Autodesk Inventor part; units mm, degrees
ref_plane "Work Plane1" through (24.6957, 5, 24.6957) normal (0.7071068, 0, 0.7071068) x (0.7071068, 0, -0.7071068)
ref_plane "YZ Plane" through (0, 0, 0) normal (1, 0, 0) x (0, 1, 0)
ref_plane "XZ Plane" through (0, 0, 0) normal (0, 1, 0) x (-1, 0, 0)
sketch "Sketch1" plane through (0, 0, 0) normal (0, 1, 0) x (-1, 0, 0)
  line L0 (101.6, -101.6) -> (-101.6, -101.6)
  line L1 (-101.6, -101.6) -> (-101.6, 101.6)
  line L2 (-101.6, 101.6) -> (101.6, 101.6)
  line L3 (101.6, 101.6) -> (101.6, -101.6)
  line L4 (96.6, -96.6) -> (-96.6, -96.6)
  line L5 (-96.6, -96.6) -> (-96.6, 96.6)
  line L6 (-96.6, 96.6) -> (96.6, 96.6)
  line L7 (96.6, 96.6) -> (96.6, -96.6)
  line L8 (101.6, 101.6) -> (-40.4, 101.6)
  circle A0 centre (0, 0) radius 88.9
  circle A1 centre (0, 0) radius 109.3376
  line L9 (-40.4, 101.6) -> (-101.6, 40.4)
  line L10 (-45.4, 101.6) -> (-101.6, 45.4)
  line L11 (96.6, 96.6) -> (96.6, 101.6)
  line L12 (-45.4, 101.6) -> (-35.4, 101.6)
  line L13 (-35.4, 101.6) -> (-35.4, 96.6)
  line L14 (-35.4, 96.6) -> (-45.4, 96.6)
  line L15 (-45.4, 96.6) -> (-45.4, 101.6)
  line L16 (-45.4, 101.6) -> (-43.114, 101.6)
  line L17 (-43.114, 101.6) -> (-43.114, 96.6)
  line L18 (-43.114, 96.6) -> (-45.4, 96.6)
  line L19 (-45.4, 96.6) -> (-45.4, 101.6)
  line L20 (-96.6, 45.4) -> (-101.6, 45.4)
  line L21 (-101.6, 45.4) -> (-101.6, 43.114)
  line L22 (-101.6, 43.114) -> (-96.6, 43.114)
  line L23 (-96.6, 43.114) -> (-96.6, 45.4)
  point P0 (96.6, 51.2168)
  point P1 (101.6, 40.4)
  point P2 (101.6, -40.4)
  point P3 (96.6, -51.2168)
  point P4 (-96.6, 45.4)
  point P5 (-45.4, 96.6)
  dimension "d0" = 203.2
  dimension "d1" = 203.2
  dimension "d2" = 101.6
  dimension "d3" = 101.6
  dimension "d4" = 5
  dimension "d5" = 5
  dimension "d6" = 5
  dimension "d7" = 5
  dimension "d10" = 142
  dimension "d12" = 61.2
  dimension "d14" = 177.8
  dimension "d15" = 5
  dimension "d16" = 5
  dimension "d17" = 10
  dimension "d86" = 2.286
  dimension "d87" = 2.286
extrude "Extrusion1" add sketch "Sketch1" along normal blind 5 contours L0 A1 L4 L7 L3 | L0 A1 L4 | A1 L7 L3 | L0 L1 A1 L5 L4 | A1 L7 L4 | L4 A1 L5 L9 L6 L7 | A1 L7 L11 L2 L3 | L4 L5 A1 | A1 L6 L7 | L1 L9 L22 L5 A1 | L11 L6 A1 L2 | L6 L13 L2 A1 | L1 L22 A1 | A1 L22 L9 | L22 L9 L5 | L6 L17 L9 L2 L13 | L1 L20 A1 L22 | A1 L20 L9 L22 | L20 A1 L10 L5 | L5 L10 L6 L9 | A1 L17 L2 | L9 L17 A1 | L6 L9 L17 | L1 L2 L10 A1 L6 L5 | L10 A1 L20 | L10 A1 L5 | L5 A1 L6 L10 | L15 A1 L17 L9 | L6 L10 A1 L15 | L17 A1 L15 L2 | L5 L6 A1 | L6 A1 L10 | A1 L10 L15 | A0
sketch "Sketch3" plane through (0, 5, 0) normal (0, 1, 0) x (1, 0, 0)
  circle A0 centre (0, 0) radius 88.9
  line L0 (-101.6, 101.6) -> (-101.6, -101.6)
  line L1 (-101.6, -101.6) -> (101.6, -101.6)
  line L2 (-101.6, 101.6) -> (101.6, 101.6)
  line L3 (101.6, 101.6) -> (101.6, -101.6)
  line L4 (101.6, -101.6) -> (-101.6, -101.6)
  line L5 (-101.6, -101.6) -> (-101.6, 101.6)
  line L6 (-96.6, 96.6) -> (96.6, 96.6)
  line L7 (96.6, 96.6) -> (96.6, -96.6)
  line L8 (96.6, -96.6) -> (-96.6, -96.6)
  line L9 (-96.6, -96.6) -> (-96.6, 96.6)
  line L10 (-101.6, -101.6) -> (40.4, -101.6)
  circle A1 centre (0, 0) radius 109.3376
  line L11 (40.4, -101.6) -> (101.6, -40.4)
  line L12 (101.6, -101.6) -> (101.6, 101.6)
  line L13 (45.4038, -101.6) -> (101.6, -45.4038)
  line L14 (96.6, -45.4) -> (101.6, -45.4038)
  line L15 (45.4, -96.6) -> (45.4038, -101.6)
  line L16 (96.6, -45.4) -> (101.6, -45.4)
  line L17 (101.6, -45.4) -> (101.6, -43.114)
  line L18 (101.6, -43.114) -> (96.6, -43.114)
  line L19 (96.6, -43.114) -> (96.6, -45.4)
  line L20 (45.4038, -101.6) -> (43.1178, -101.6)
  line L21 (43.1178, -101.6) -> (43.1178, -96.6)
  line L22 (43.1178, -96.6) -> (45.4038, -96.6)
  line L23 (45.4038, -96.6) -> (45.4038, -101.6)
  point P0 (45.4038, -101.6)
  point P1 (50.4038, -96.6)
  point P2 (96.6, -50.4038)
  dimension "d28" = 177.8
  dimension "d29" = 5
  dimension "d30" = 5
  dimension "d31" = 5
  dimension "d32" = 5
  dimension "d33" = 142
  dimension "d76" = 5.0038
  dimension "d77" = 5.0038
  dimension "d88" = 2.286
  dimension "d89" = 2.286
extrude "Extrusion3" cut sketch "Sketch3" against normal blind 2 contours L2 A1 L6 L9 L0 | A1 L9 L0 | L2 A1 L6 | A1 L9 L8 L1 L0 | L2 L3 A1 L7 L6 | A1 L8 L21 L11 L1 | L3 L11 L18 L7 A1 | A1 L21 L1 | L11 L21 A1 | L3 L18 A1 | A1 L18 L11
sketch "Sketch4" plane through (0, 5, 0) normal (0, 1, 0) x (1, 0, 0)
  line L0 (101.6, 101.6) -> (-101.6, 101.6)
  line L1 (-101.6, 101.6) -> (-101.6, -101.6)
  line L2 (-101.6, -101.6) -> (101.6, -101.6)
  line L3 (101.6, -101.6) -> (101.6, 101.6)
  circle A0 centre (0, 0) radius 2.5
  line L4 (11.3314, 2.139) -> (-2.139, -11.3314)
  line L5 (0, 0) -> (-5.6569, 5.6569)
  line L6 (-5.6569, -14.8492) -> (-26.163, 5.6569)
  line L7 (-5.6569, 26.163) -> (14.8492, 5.6569)
  circle A1 centre (-5.6569, 5.6569) radius 14
  line L8 (-26.163, 5.6569) -> (-5.6569, 26.163)
  line L9 (14.8492, 5.6569) -> (-5.6569, -14.8492)
  line L10 (-40.3051, 5.6569) -> (-5.6569, 40.3051)
  line L11 (-5.6569, 40.3051) -> (28.9914, 5.6569)
  line L12 (28.9914, 5.6569) -> (-5.6569, -28.9914)
  line L13 (-5.6569, -28.9914) -> (-40.3051, 5.6569)
  line L14 (-22.6451, 9.1747) -> (-9.1747, 22.6451)
  line L15 (-9.1747, 22.6451) -> (-12.7668, 26.2372)
  line L16 (-12.7668, 26.2372) -> (-26.2372, 12.7668)
  line L17 (-26.2372, 12.7668) -> (-22.6451, 9.1747)
  point P0 (9.525, 22.5)
  point P1 (-9.525, -6.5)
  dimension "d37" = 203.2
  dimension "d38" = 203.2
  dimension "d39" = 8
  dimension "d40" = 28
  dimension "d41" = 29
  dimension "d42" = 29
  dimension "d43" = 14.5
  dimension "d44" = 10
  dimension "d45" = 10
  dimension "d46" = 10
  dimension "d47" = 10
  dimension "d48" = 5.08
  dimension "d49" = 9.525
  dimension "d50" = 9.525
  dimension "d55" = 101.6
  dimension "d56" = 101.6
extrude "Extrusion4" cut sketch "Sketch4" against normal blind 1 contours A0 | L4 L9 L6 L8 L7 | L8 L17 L16 L15 | A1 | L10 L11 L12 L13
sketch "Sketch6" plane through (0, 5, 0) normal (0, 1, 0) x (1, 0, 0)
  line L0 (45.4038, -101.6) -> (0, 0)
  line L1 (50.4038, -96.6) -> (45.4038, -101.6)
  line L2 (96.6, -43.114) -> (96.6, 96.6)
  line L3 (101.6, -101.6) -> (101.6, 101.6)
  circle A0 centre (0, 0) radius 34.925
  circle A1 centre (0, 0) radius 33.425
  line L4 (-101.6, 101.6) -> (-101.6, -101.6)
  line L5 (-101.6, -101.6) -> (40.4, -101.6)
  line L6 (-101.6, -101.6) -> (101.6, -101.6)
  line L7 (101.6, 101.6) -> (101.6, -43.114)
  line L8 (101.6, -45.4038) -> (0, 0)
  line L9 (-96.6, -96.6) -> (43.1178, -96.6)
  line L10 (96.6, -43.114) -> (96.6, 96.6)
  line L11 (43.1178, -101.6) -> (-101.6, -101.6)
  line L12 (101.6, -45.4038) -> (96.6, -50.4038)
  line L13 (45.4038, -101.6) -> (101.6, -45.4038)
  line L14 (43.1178, -101.6) -> (101.6, -101.6)
  line L15 (0, 0) -> (101.6, -50.4076)
  line L16 (50.4076, -101.6) -> (0, 0)
  line L17 (43.1694, -96.6) -> (47.9269, -96.6)
  line L18 (96.6, -43.1694) -> (96.6, -47.9269)
  line L19 (40.4, -101.6) -> (101.6, -40.4)
  point P0 (13.6374, -30.5164)
  point P1 (30.5164, -13.6374)
  point P2 (14.2494, -31.8859)
  point P3 (31.2861, -15.5222)
  point P4 (29.9423, -14.8555)
  point P5 (31.8859, -14.2494)
  point P6 (98.2555, -48.7483)
  point P7 (96.6, -47.9269)
  point P8 (47.9269, -96.6)
  point P9 (15.5222, -31.2861)
  point P10 (96.6, -45.4)
  point P11 (45.4, -96.6)
  point P12 (14.8555, -29.9423)
  point P13 (96.6, -45.4)
  point P14 (45.4, -96.6)
  point P15 (45.4, -96.6)
  point P16 (47.089, -94.911)
  point P17 (94.911, -47.089)
  point P18 (96.6, -45.4)
  point P19 (43.8583, -98.1417)
  point P20 (98.1417, -43.8583)
  point P21 (45.4, -96.6)
  point P22 (96.6, -45.4)
  dimension "d71" = 69.85
  dimension "d72" = 66.85
  dimension "d75" = 142
  dimension "d78" = 5.0038
  dimension "d82" = 5.0038
extrude "Extrusion6" add sketch "Sketch6" along normal blind 54.5 contours L0 A0 L16 L19 L17 | L0 A1 L16 A0 | L16 A1 L15 A0 | L15 A0 L8 L18 L19 | A0 L15 A1 L8
fillet "Fillet3" radius 12.7 1 edges at (101.6, 2.5, 101.6)
sketch "Sketch9" plane through (0, 4, 0) normal (0, 1, 0) x (1, 0, 0)
  point P0 (0, 0)
sketch "Sketch10" plane through (0, 5, 0) normal (0, 1, 0) x (1, 0, 0)
  point P0 (0, 0)
ref_plane "Work Plane1" through (24.6957, 5, 24.6957) normal (0.7071068, 0, 0.7071068) x (0.7071068, 0, -0.7071068)
sketch "Sketch15" plane through (0, 5, 0) normal (0, 1, 0) x (1, 0, 0)
  line L0 (13.6374, -30.5164) -> (43.1694, -96.6)
  line L1 (28.4034, -63.5582) -> (-0.6569, -23.9914)
  line L2 (28.9914, 5.6569) -> (-5.6569, -28.9914)
  line L3 (96.6, -43.1694) -> (30.5164, -13.6374)
  line L4 (-5.6569, 40.3051) -> (28.9914, 5.6569)
  line L5 (63.5582, -28.4034) -> (23.9914, 0.6569)
  line L6 (2.3374, -28.0682) -> (28.0682, -2.3374)
  arc A0 (13.6374, -30.5164) -> (30.5164, -13.6374) centre (0, 0) ccw
  line L7 (28.4034, -63.5582) -> (13.6374, -30.5164)
  line L8 (63.5582, -28.4034) -> (30.5164, -13.6374)
  arc A1 (13.6374, -30.5164) -> (30.5164, -13.6374) centre (0, 0) ccw
  dimension "d138" = 5
  dimension "d139" = 5
  dimension "d140" = 5
extrude "Extrusion11" add sketch "Sketch15" along normal up to surface (54.5 mm away) contours L0 L1 L6 L5 L3 A0
sketch "Sketch16" plane through (0, 59.5, 0) normal (0, 1, 0) x (1, 0, 0)
  line L0 (2.3374, -28.0682) -> (28.0682, -2.3374)
  line L1 (9.4085, -20.9971) -> (12.944, -24.5327)
  line L2 (12.944, -24.5327) -> (24.5327, -12.944)
  line L3 (24.5327, -12.944) -> (20.9971, -9.4085)
  line L4 (12.944, -24.5327) -> (24.5327, -12.944)
  line L5 (24.5327, -12.944) -> (28.5592, -16.9706)
  line L6 (28.5592, -16.9706) -> (16.9706, -28.5592)
  line L7 (16.9706, -28.5592) -> (12.944, -24.5327)
  line L8 (12.944, -24.5327) -> (5.3317, -32.145)
  line L9 (28.4034, -63.5582) -> (2.3374, -28.0682)
  line L10 (24.5327, -12.944) -> (32.145, -5.3317)
  line L11 (28.0682, -2.3374) -> (63.5582, -28.4034)
  point P0 (0, 0)
  dimension "d144" = 10
  dimension "d145" = 10
  dimension "d146" = 5
  dimension "d152" = 0
  dimension "d153" = 0
extrude "Extrusion12" cut sketch "Sketch16" against normal up to surface (54.5 mm away)
sketch "Sketch11" plane through (24.6957, 5, 24.6957) normal (0.7071068, 0, 0.7071068) x (0.7071068, 0, -0.7071068)
  line L0 (143.6841, -5) -> (0, -5)
  line L1 (0, -5) -> (0, 26.75)
  circle A0 centre (0, 26.75) radius 5.5
  line L2 (0, 26.75) -> (0, 45.8)
  circle A1 centre (0, 45.8) radius 3
  dimension "d120" = 31.75
  dimension "d121" = 11
  dimension "d171" = 19.05
  dimension "d172" = 6
extrude "Extrusion8" cut sketch "Sketch11" against normal blind 127
sketch "Sketch17" plane through (5.3317, 5, 32.145) normal (-0.7071068, 0, -0.7071068) x (-0.7071068, 0, 0.7071068)
  circle A0 centre (-29.4679, 45.7716) radius 1.1146
  circle A1 centre (-8.4493, 45.7716) radius 1.1245
  circle A2 centre (-8.4493, 33.2324) radius 1.229
  circle A3 centre (-29.4679, 33.2324) radius 1.2635
  line L0 (-29.4679, 45.7716) -> (-8.4493, 45.7716)
  line L1 (-8.4493, 45.7716) -> (-8.4493, 33.2324)
  line L2 (-8.4493, 33.2324) -> (-29.4679, 33.2324)
  line L3 (-29.4679, 33.2324) -> (-29.4679, 45.7716)
  line L4 (-24.4164, 38.6993) -> (-13.5188, 38.6993)
  line L5 (-13.5188, 38.6993) -> (-13.5188, 27.7864)
  line L6 (-13.5188, 27.7864) -> (-24.4164, 27.7864)
  line L7 (-24.4164, 27.7864) -> (-24.4164, 38.6993)
  line L8 (-31.5058, 47.9379) -> (-6.5058, 47.9379)
  line L9 (-6.5058, 47.9379) -> (-6.5058, 23.4716)
  line L10 (-6.5058, 23.4716) -> (-31.5058, 23.4716)
  line L11 (-31.5058, 23.4716) -> (-31.5058, 47.9379)
  line L12 (-18.9599, -5) -> (-18.9599, 33.1)
  point P0 (-29.4871, 46.9004)
  point P1 (-8.4871, 46.9004)
  point P2 (-8.3009, 35.9211)
  point P3 (-29.3009, 35.902)
  dimension "d185" = 21.0186
  dimension "d186" = 12.5392
  dimension "d187" = 2.249
  dimension "d188" = 25
  dimension "d189" = 24.4663
  dimension "d190" = 38.1
  dimension "d191" = 5.4565
  dimension "d192" = 5.4411
hole "Hole1" at (26.1822, 51.9004, 11.2945) at (26.0505, 40.902, 11.4261) at (11.3329, 51.9004, 26.1437) at (11.2013, 40.9211, 26.2754) direction (0.7071068, 0, 0.7071068) diameter 2.85 depth 5.08 tip angle 118 countersink diameter 3.048 countersink angle 82
sketch "Sketch18" plane through (101.6, 3, 43.114) normal (1, 0, 0) x (0, 0, -1)
  line L0 (-53.486, 2) -> (-58.486, 2)
  line L1 (-58.486, 2) -> (145.4353, 2)
  line L2 (145.4353, 2) -> (145.4353, -4.8825)
  line L3 (145.4353, -4.8825) -> (-58.486, -4.8825)
  line L4 (-58.486, -4.8825) -> (-58.486, 2)
  point P0 (43.114, -3)
extrude "Extrusion13" cut sketch "Sketch18" against normal through all
sketch "Sketch21" plane through (0, 59.5, 0) normal (0, 1, 0) x (1, 0, 0)
  line L0 (0, 0) -> (73.3665, -73.3665)
  line L1 (0, 0) -> (103.756, 0) construction
  dimension "d173" = 45
equation "\"d1\" = d0"
properties part number "Box_Walls_2"
Read the model definition and answer for the solid it produces. Units are mm, in the model's axes. A direction names the side the tool comes from. Coordinates: 2 decimals unless noted, no trailing zeros. Write each loop counter-clockwise with the first axis right and the second up, starting at its lowest first coordinate (ties: lowest second). Pieces come first, ordered by that corner, then holes. Notation, with made-up numbers: (-17, -33) -> (10, -33) arc R14 cw to (10, -14) -> close; hole circle Ø3 at (74, 82). An arc over 180 degrees is marked (long way). Return JSON: item names as keys, results as strings.
1. A cutting plane is placed at B-B (z = 35). Determine the outline of the cut face in (x, y).
Found:
{"outline": "(7.43, 5) -> (17.36, 5) -> (17.36, 59.5) -> (7.43, 59.5) -> close; (70.54, 5) -> (78.32, 5) -> (78.32, 59.5) -> (70.54, 59.5) -> close"}
2. A cutting plane is placed at C-C (y = 16.5). Determine the outline of the cut face in (x, z) (3 decimals), and give its area (3 significant figures).
Found:
{"outline": "(5.332, 32.145) -> (12.944, 24.533) -> (16.971, 28.559) -> (28.559, 16.971) -> (24.533, 12.944) -> (32.145, 5.332) -> (63.558, 28.403) -> (96.6, 43.169) -> (96.6, 45.4) -> (94.911, 47.089) -> (31.286, 15.522) arc R34.925 ccw to (15.522, 31.286) -> (47.089, 94.911) -> (45.4, 96.6) -> (43.169, 96.6) -> (28.403, 63.558) -> close", "area": "830 mm2"}
3. Find the intervals of material crossed by line 1 along Z through (x, y) = (35, 16); line 2 along X through (y, z) = (22.5, 28); line 3 along Z through (x, y) = (17, 29), in increasing order. Write a range as from..to.
Found:
{"line 1": "7.43..17.36, 70.54..78.32", "line 2": "9.48..16.41, 17.53..20.87, 56.44..63.01", "line 3": "28.53..30.51, 34.26..48.03"}
4. Determine the mould class of faces 4 (the face through (44, 5, 21)), 5 (the face through (28.656, 50.77, 12.542)), 6 (the face through (27.45, 33.4, 20.03)), 7 (the face through (48.07, 31.87, 17.03)) for opening direction Y: pulls with the +Y half, pulls with the -Y half, needs draft (parallel to the pull), parting line crosses it, or undercut.
Found:
{"face 4": "pulls with the -Y half", "face 5": "undercut", "face 6": "undercut", "face 7": "needs draft"}
5. Each of these flat-tipped pins is pushed along its axis until it touches: P1, Ø5, axis at y = 13, z = 54, coming from the +X side; P2, Ø4, axis at y = 16, z = 84.5, coming from the -X side; P3, Ø3, axis at x = 73.5, y = 33.5, coming from the -Z side. Where does it stop, or does it pass through?
Found:
{"P1": "x = 28.03", "P2": "x = 36.87", "P3": "z = 32.18"}
6. A cutting plane is placed at D-D (x = 78). Determine the outline of the cut face in (y, z).
Found:
{"outline": "(5, 34.86) -> (59.5, 34.86) -> (59.5, 38.7) -> (5, 38.7) -> close"}
7. A cutting plane is placed at A-A (y = 49). Determine the outline of the cut face in (x, z) (3 decimals).
Found:
{"outline": "(5.332, 32.145) -> (12.944, 24.533) -> (16.971, 28.559) -> (21.068, 24.462) -> (22.94, 26.334) arc R34.925 ccw to (15.522, 31.286) -> (47.089, 94.911) -> (45.4, 96.6) -> (43.169, 96.6) -> (28.403, 63.558) -> close; (24.462, 21.068) -> (28.559, 16.971) -> (24.533, 12.944) -> (32.145, 5.332) -> (63.558, 28.403) -> (96.6, 43.169) -> (96.6, 45.4) -> (94.911, 47.089) -> (31.286, 15.522) arc R34.925 ccw to (26.334, 22.94) -> close"}
8. A tool of negligible diameter and unlimited length cuts with its end or side. For faces 1 (the face through (14.985, 32.632, 26.574)), 2 (the face through (13.448, 42.237, 27.75)), 3 (the face through (25.42, 26.58, 20.11)), from which of +Z, -Z, +X, -X, +Y, -Y can it reach the whole face along a straight path? Write none if from no direction.
Found:
{"face 1": "-Z, +Y, -Y", "face 2": "none", "face 3": "+Y, -Y"}
